Design review of the part built by this model. Coordinates are the model's own, in mm. Give positions to 0.01 mm unless a question says otherwise; leave off trailing zeros. Order: outer loops, then holes, each group sorted by start corner. A loop starts at its lowest first (then second) coordinate and runs counter-clockwise, first axis right, second up. Notation, with made-up numbers: M 28.25,61 L 36.25,61 A14 cw 36.25,70 Z; hole C 18,61.5 d2. An arc over 180 degrees is marked long. Answer as a JSON object with one key per item and string values.
from build123d import *

# Parameters (mm, degrees)
F0_R     = 5
F0_R_2   = 4
F1_DEPTH = 6.8
F2_SIZE  = 0.2
F3_SIZE  = 0.2
F4_SIZE  = 0.2


with BuildPart() as f1:
    # F0 (on Top) → F1 (new body)
    with BuildSketch(Plane.XY):
        Circle(F0_R)
        Circle(F0_R_2, mode=Mode.SUBTRACT)
    extrude(amount=F1_DEPTH)

    # F2
    f2_edges = [f1.edges().sort_by_distance(p)[0] for p in [
        (-4, 0, 6.8),
    ]]
    chamfer(f2_edges, length=F2_SIZE)

    # F3
    f3_edges = [f1.edges().sort_by_distance(p)[0] for p in [
        (-5, 0, 6.8),
    ]]
    chamfer(f3_edges, length=F3_SIZE)

    # F4
    f4_edges = [f1.edges().sort_by_distance(p)[0] for p in [
        (-5, 0, 0),
        (-4, 0, 0),
    ]]
    chamfer(f4_edges, length=F4_SIZE)


solid = f1.part
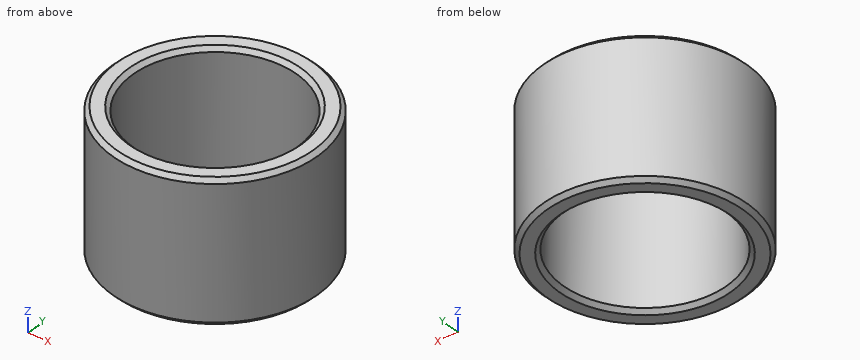
(1) We need section A-A (y = 0). Write out the cut boundary in (x, z).
Checked values:
{"outline": "M -5,0.2 L -4.8,0 L -4.2,0 L -4,0.2 L -4,6.6 L -4.2,6.8 L -4.8,6.8 L -5,6.6 Z; M 4,0.2 L 4.2,0 L 4.8,0 L 5,0.2 L 5,6.6 L 4.8,6.8 L 4.2,6.8 L 4,6.6 Z"}
(2) To check wall thickness, follow L1, parallel to Y at x = 0, z = 2; L2, parallel to X at y = -1.5, z = 2.25; L3, parallel to Y at x = -3, z = 1.25. State the ranges of each line that lie inside material, in increasing order. Write a range as from..to.
Checked values:
{"L1": "y = -5..-4, 4..5", "L2": "x = -4.77..-3.71, 3.71..4.77", "L3": "y = -4..-2.65, 2.65..4"}
(3) Insertion check: pin 1 (6 mm diameter, centred on x = -2, y = 2, fed in from +Z); pin 2 (1 mm diameter, centred on y = -1, z = 3.5, fed in from -X); pin 3 (1.5 mm diameter, centred on y = 2, z = 4, fed in from -X). Each pin has a flat end and moves straight along its axis. Give the tip position at first contact, or say it passes through.
Checked values:
{"pin 1": "stops at z = 6.8", "pin 2": "stops at x = -4.97", "pin 3": "stops at x = -4.84"}
(4) We need section C-C (z = 3.75). Write out the cut boundary in (x, y), plus the area to 3 significant figures.
Checked values:
{"outline": "C 0,0 d10; hole C 0,0 d8", "area": "28.3 mm^2"}
